```python
from build123d import *

# Parameters (mm, degrees)
SKETCH1_W                   = 25.4
SKETCH1_H                   = 25.4
SKETCH1_W_2                 = 22.225
SKETCH1_H_2                 = 22.225
BOSS_EXTRUDE1_DEPTH         = 487.68
F_1_4_0_25_DIAMETER_HOLE1_D = 6.35


with BuildPart() as part:
    # Sketch1 → Boss-Extrude1 (new body)
    with BuildSketch(Plane(origin=(0, 0, 0), x_dir=(1, 0, 0), z_dir=(0, 1, 0))):
        Rectangle(SKETCH1_W, SKETCH1_H)
        Rectangle(SKETCH1_W_2, SKETCH1_H_2, mode=Mode.SUBTRACT)
    extrude(amount=BOSS_EXTRUDE1_DEPTH)

    # 1/4 (0.25) Diameter Hole1 (through all)
    with Locations(Plane.XY.offset(12.7)):
        with Locations((0, 474.98), (0, 292.1)):
            Hole(F_1_4_0_25_DIAMETER_HOLE1_D / 2)


solid = part.part
```
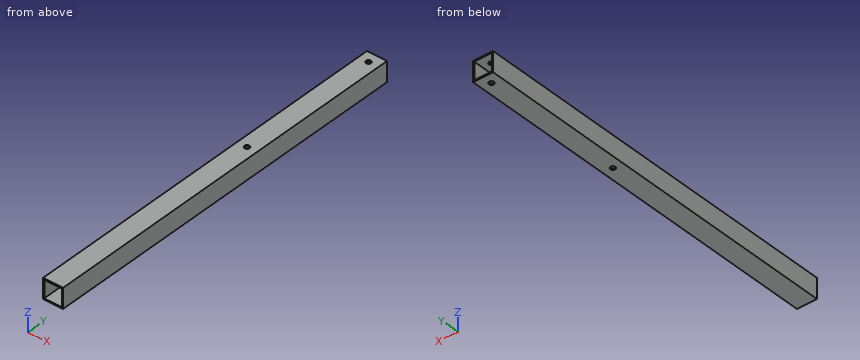
Geometry: final body of the model. Coordinates: model frame, mm. Coordinates: 2 decimals unless noted, no trailing zeros. Loops run counter-clockwise (first coordinate to the right, second up) from the corner with the lowest first, then second, coordinate; pieces in that order, holes last. Notation, with made-up numbers: (65.5, 32.25) -> (90.5, 32.25) arc R3 ccw to (90.5, 37.25) -> close; hole circle Ø1 at (38.25, 13.25). An arc over 180 degrees is marked (long way). Use a Markdown table: item, result. Add a question column.
(1) Section query A-A, the plane z = 3. Return loops of the section in (x, y).
(2) Section query C-C, the plane y = 394.5. Return loops of the section in (x, z), plus the area to 3 significant figures.
(3) Line query: line 1 along Y through (x, z) = (0, -11.9) (3 decimals); line 2 along X through (y, z) = (301, -4); line 3 along X through (y, z) = (474.98, -11.9) (3 decimals). Output: solid intervals per line, ascending.
(4) Section query B-B, the plane x = 7. Return loops of the section in (y, z).
Answer:
| question | item | result |
|---|---|---|
| 1 | outline | (-12.7, 0) -> (-11.11, 0) -> (-11.11, 487.68) -> (-12.7, 487.68) -> close; (11.11, 0) -> (12.7, 0) -> (12.7, 487.68) -> (11.11, 487.68) -> close |
| 2 | outline | (-12.7, -12.7) -> (12.7, -12.7) -> (12.7, 12.7) -> (-12.7, 12.7) -> close; hole (-11.11, -11.11) -> (11.11, -11.11) -> (11.11, 11.11) -> (-11.11, 11.11) -> close |
| 2 | area | 151 mm^2 |
| 3 | line 1 | y = 0 to 288.925, 295.275 to 471.805, 478.155 to 487.68 |
| 3 | line 2 | x = -12.7 to -11.11, 11.11 to 12.7 |
| 3 | line 3 | x = -12.7 to -3.175, 3.175 to 12.7 |
| 4 | outline | (0, -12.7) -> (487.68, -12.7) -> (487.68, -11.11) -> (0, -11.11) -> close; (0, 11.11) -> (487.68, 11.11) -> (487.68, 12.7) -> (0, 12.7) -> close |
